Autodesk Inventor part; units mm, degrees
ref_plane "YZ Plane" through (0, 0, 0) normal (1, 0, 0) x (0, 1, 0)
ref_plane "XZ Plane" through (0, 0, 0) normal (0, 1, 0) x (-1, 0, 0)
ref_plane "XY Plane" through (0, 0, 0) normal (0, 0, 1) x (1, 0, 0)
sketch "Sketch1" plane through (0, 0, 0) normal (0, 1, 0) x (-1, 0, 0)
  line L0 (0, 0) -> (20, 0)
  line L1 (20, 0) -> (20, -20)
  line L2 (20, -20) -> (0, -20)
  line L3 (0, -20) -> (0, 0)
  dimension "d0" = 20
  dimension "d1" = 20
extrude "Extrusion1" add sketch "Sketch1" along normal blind 3
sketch "Sketch2" plane through (0, 3, 0) normal (0, 1, 0) x (1, 0, 0)
  circle A0 centre (-10, 15) radius 3
  line L0 (0, 0) -> (0, 20)
  line L1 (0, 20) -> (-20, 20)
  circle A1 centre (-10, 5) radius 3
  dimension "d4" = 6
  dimension "d5" = 10
  dimension "d6" = 5
  dimension "d23" = 6
  dimension "d24" = 10
  dimension "d25" = 10
extrude "Extrusion2" cut sketch "Sketch2" against normal through all
sketch "Sketch3" plane through (0, 3, 0) normal (0, 1, 0) x (1, 0, 0)
  circle A0 centre (-10, 15) radius 3
  circle A1 centre (-10, 15) radius 5
  line L0 (-10, 15) -> (-18, 15)
  line L1 (0, 20) -> (-20, 20)
  line L2 (-20, 0) -> (-16, 0)
  line L3 (-16, 0) -> (-16, 20)
  line L4 (-16, 20) -> (-20, 20)
  line L5 (-20, 20) -> (-20, 0)
  line L6 (0, 0) -> (0, 20)
  dimension "d9" = 10
  dimension "d10" = 8
  dimension "d11" = 4
  dimension "d26" = 20
  dimension "d27" = 20
extrude "Extrusion3" add sketch "Sketch3" along normal blind 17 contours L3 L2 L5 L1
sketch "Sketch4" plane through (-20, 0, -20) normal (-1, 0, 0) x (0, 0, 1)
  line L0 (0, 0) -> (0, 20)
  line L1 (0, 20) -> (20, 20)
  line L2 (20, 20) -> (20, 18)
  line L3 (20, 18) -> (0, 18)
  line L4 (0, 18) -> (0, 20)
  point P0 (20, 0)
  dimension "d14" = 20
  dimension "d15" = 2
extrude "Extrusion4" add sketch "Sketch4" along normal blind 4
fillet "Fillet1" radius 2 1 edges at (-16, 20, -10)
fillet "Fillet2" radius 2 1 edges at (-20, 18, -10)
fillet "Fillet3" radius 2 1 edges at (-20, 0, -10)
fillet "Fillet4" radius 2 1 edges at (-16, 3, -10)
fillet "Fillet5" radius 2 2 edges at (0, 3, -10) (0, 0, -10)
properties part number "CableGuide"
Input: part model. Units: mm. Frame: model coordinates. A direction names the side the tool comes from. Coordinates: 2 decimals unless noted, no trailing zeros. Order: outer loops, then holes, each group sorted by start corner. A loop starts at its lowest first (then second) coordinate and runs counter-clockwise, first axis right, second up. Notation, with made-up numbers: M 30,29 L 57,29 A28 ccw 57,62 Z; hole C 16,55.5 d11. An arc over 180 degrees is marked long. Write item = value, one per line. Start each with the question number.
(1) Pull-direction query (X, two-part tool) for faces 1 (the cylindrical face through (-10.65, 1.52, -12.07)), 2 (the cylindrical face through (-19.4, 0.57, -10.14)), 3 (the cylindrical face through (-15.4, 3.57, -10.14)); classes: released by +X, released by -X, zero draft, split by the parting line, or undercut.
(2) First-contact query: P1, Ø10.5, axis at y = 12, z = -8, coming from the +X side; P2, Ø3, axis at x = -14, y = 6.5, coming from the +Z side; P3, Ø1, axis at x = -23, z = -6.5, coming from the -Y side; P4, Ø2, axis at x = -3, z = -5, coming from the -Y side. Flat tips, straight axial feed; report the tip coordinate or a pass-through.
(3) Section D-D on y = 1.5. Output: boundary loops of the cut face in (x, z), and give its area (3 significant figures).
(4) Reachability of faces 4 (the flat face through (-16, 11, -10)), 5 (the cylindrical face through (-12.4, 1.5, -3.2)), 6 (the flat face through (-20, 9, -10)) from +Z, -Z, +X, -X, +Y, -Y: full face, straight path, thin tool, end or side. Return the list, or none.
(5) Section C-C on z = -1.5. Output: boundary loops of the cut face in (x, y), and give its area (3 significant figures).
(6) Section A-A on x = -10. Output: boundary loops of the cut face in (y, z), and give its area (3 significant figures).
(7) Section B-B on z = -5. Output: boundary loops of the cut face in (x, y), and give its area (3 significant figures).
(8) Line query: line 1 along Z through (x, y) = (-10, 1); line 2 along Y through (x, z) = (-11.75, -2.25); line 3 along X through (y, z) = (14.5, -8.5). Output: solid intervals per line, ascending. Write a range as [from, to].
Result set:
q1.face_1 = undercut
q1.face_2 = released by -X
q1.face_3 = released by +X
q2.P1 = -16
q2.P2 = through
q2.P3 = 18
q2.P4 = 0
q3.outline = M -19.94,-20 L -0.06,-20 L -0.06,0 L -19.94,0 Z; hole C -10,-15 d6; hole C -10,-5 d6
q3.area = 341 mm²
q4.face_4 = +Z, -Z, +X, +Y
q4.face_5 = +Y, -Y
q4.face_6 = +Z, -Z, -X, -Y
q5.outline = M -24,18 L -22,18 A2 cw -20,16 L -20,2 A2 ccw -18,0 L -1.73,0 A2 ccw 0,1 A2 ccw -2,3 L -14,3 A2 cw -16,5 L -16,18 A2 ccw -18,20 L -24,20 Z
q5.area = 135 mm²
q6.outline = M 0,-20 L 3,-20 L 3,-18 L 0,-18 Z; M 0,-12 L 3,-12 L 3,-8 L 0,-8 Z; M 0,-2 L 3,-2 L 3,0 L 0,0 Z
q6.area = 24.0 mm²
q7.outline = M -24,18 L -22,18 A2 cw -20,16 L -20,2 A2 ccw -18,0 L -13,0 L -13,3 L -14,3 A2 cw -16,5 L -16,18 A2 ccw -18,20 L -24,20 Z; M -7,0 L -1.73,0 A2 ccw 0,1 A2 ccw -2,3 L -7,3 Z
q7.area = 117 mm²
q8.line_1 = [-20, -18], [-12, -8], [-2, 0]
q8.line_2 = [0, 3]
q8.line_3 = [-20, -16]
